Here's the drawing with two shaded views (mm, measured from the low corner). I have some questions. A direction names the side the tool comes from. Round coordinates to 2 decimals unless told otherwise and drop trailing zeros. Order: outer loops, then holes, each group sorted by start corner. A loop starts at its lowest first (then second) coordinate and runs counter-clockwise, first axis right, second up. Notation, with made-up numbers: (23.5, 24) - (80.5, 24) arc R13 cw to (80.5, 48) - close; hole circle Ø9 at (86, 66). An arc over 180 degrees is marked (long way). One line per item, written item: value.
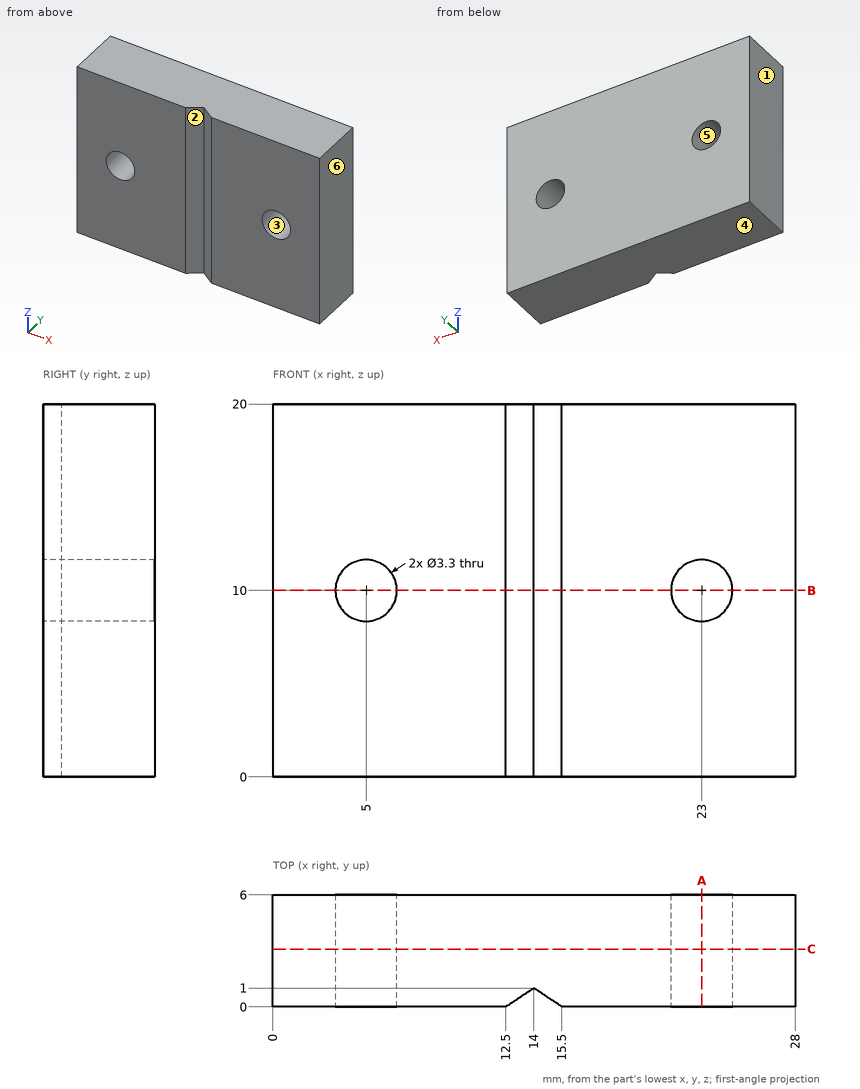
Q1. Which directions (+Z, -Z, +X, -X, +Y, -Y) give clear straight access to the entire face, cutting with the end or side of a thin tool? Please do the marked faces 1 and 2.
Results list:
face 1: +Z, -Z, -X, +Y, -Y
face 2: +Z, -Z, -Y
Q2. If we section it at C-C, the plane y = 3.1: Please give me the cut outline in (x, z), then the cut area to 3 significant figures.
Results list:
outline: (0, 0) - (28, 0) - (28, 20) - (0, 20) - close; hole circle Ø3.3 at (5, 10); hole circle Ø3.3 at (23, 10)
area: 543 mm²
Q3. If we section it at A-A, the plane x = 23: Please give me the cut outline in (y, z), then the cut area to 3 significant figures.
Results list:
outline: (0, 0) - (6, 0) - (6, 8.35) - (0, 8.35) - close; (0, 11.65) - (6, 11.65) - (6, 20) - (0, 20) - close
area: 100 mm²
Q4. We'd pull the mould along Z, two halves only. Please class the marked faces 3, 4, 5 and 6: released by +Z, released by -Z, zero draft, split by the parting line, or undercut.
Results list:
face 3: undercut
face 4: released by -Z
face 5: undercut
face 6: zero draft
Q5. If we section it at B-B, the plane z = 10: Please give me the cut outline in (x, y), then the cut area to 3 significant figures.
Results list:
outline: (0, 0) - (3.35, 0) - (3.35, 6) - (0, 6) - close; (6.65, 0) - (12.5, 0) - (14, 1) - (15.5, 0) - (21.35, 0) - (21.35, 6) - (6.65, 6) - close; (24.65, 0) - (28, 0) - (28, 6) - (24.65, 6) - close
area: 127 mm²
Q6. Will these pins go through, and if not, where does the flat tip stop? pin 1 (5.5 mm diameter, centred on x = 5, z = 10, fed in from +Y); pin 2 (2 mm diameter, centred on x = 23, z = 10, fed in from +Y).
Results list:
pin 1: y = 6
pin 2: through
Q7. If I drill on line 1 along Z through (x, y) = (5, 3.85); line 2 along X through (y, z) = (0.75, 8) (3 decimals); line 3 along Z through (x, y) = (24.5, 0.95), over which ranges is the centre line in solid material (lowest first)?
Results list:
line 1: 0 to 8.35, 11.65 to 20
line 2: 0 to 13.625, 14.375 to 28
line 3: 0 to 9.31, 10.69 to 20
